Design review of the part shown in the three views and the two pictorial views. Dimensions are in mm from the part's minimum x, y and z. A direction names the side the tool comes from. Round coordinates to 2 decimals unless told otherwise and drop trailing zeros. Order: outer loops, then holes, each group sorted by start corner. A loop starts at its lowest first (then second) coordinate and runs counter-clockwise, first axis right, second up. Notation, with made-up numbers: M 84,87.5 L 101,87.5 A19 ccw 101,96.5 Z; hole C 15,-35.75 d9. An arc over 180 degrees is marked long. Write item = value, one per line. Start each with the question number.
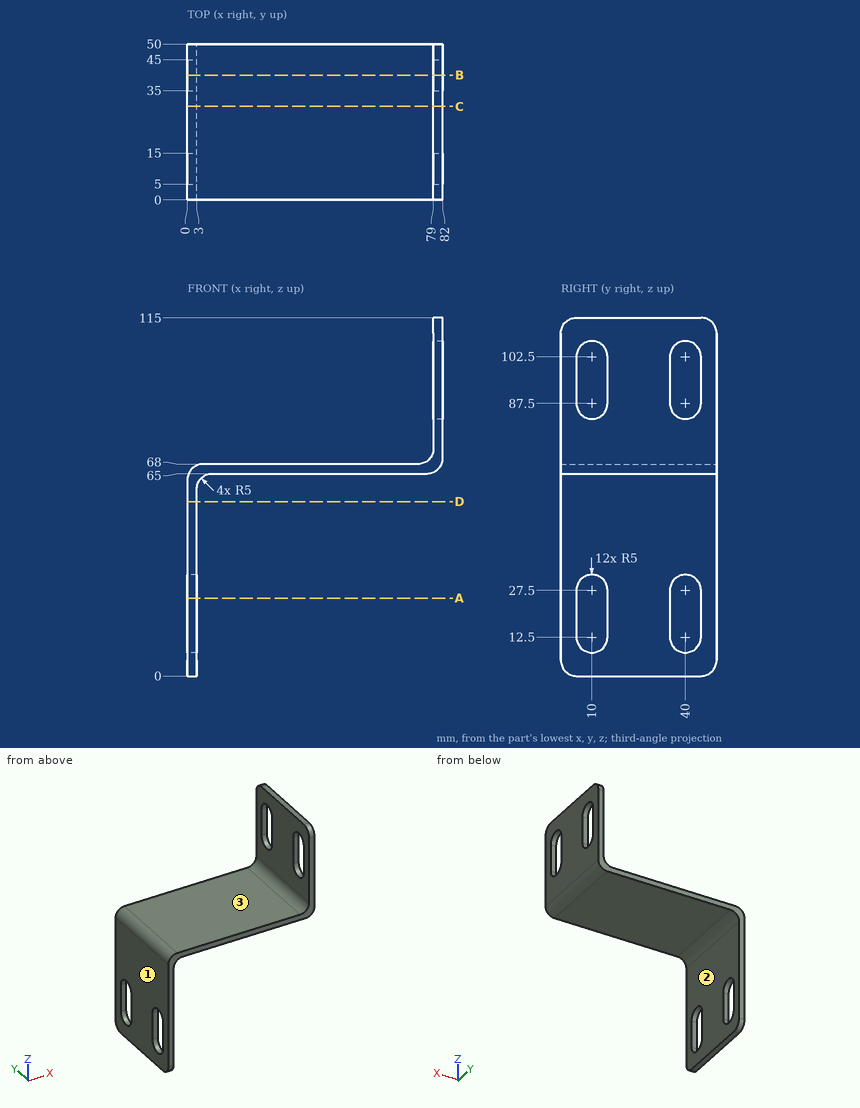
(1) For the marked faces 1, 2 and 3, list the 3-axis set-ups (+Z, -Z, +X, -X, +Y, -Y) from which the entire face can be reached by the end or side of a thin tool; tool diameter is ignored.
(2) For line 1 along X through (y, z) = (36, 41); line 2 along Z through (x, y) = (43.5, 47.5); line 3 along X through (y, z) = (31.5, 83), list the stretches that pass through material, from the lowest coordinate up.
(3) We need section B-B, the plane y = 40. Write out the cut boundary in (x, z).
(4) We need section A-A, the plane z = 25. Write out the cut boundary in (x, y), then the cut area to 3 significant figures.
(5) We need section D-D, the plane z = 56. Write out the cut boundary in (x, y).
(6) We need section C-C, the plane y = 30. Write out the cut boundary in (x, z), then the cut area to 3 significant figures.
(7) Insertion check: pin 1 (3 mm diameter, centred on x = 58, y = 6.5, fed in from +Z); pin 2 (15 mm diameter, centred on x = 48.5, y = 15, fed in from -Z); pin 3 (8 mm diameter, centred on y = 7, z = 99, fed in from -X). Each pin has a flat end and moves straight along its axis. Give the tip position at first contact, or say it passes through.
Values:
q1.face_1 = +Z, -Z, -X, +Y, -Y
q1.face_2 = -Z, +X, +Y, -Y
q1.face_3 = +Z, -X, +Y, -Y
q2.line_1 = 0 to 3
q2.line_2 = 65 to 68
q2.line_3 = 79 to 82
q3.outline = M 0,0 L 3,0 L 3,7.5 L 0,7.5 Z; M 0,32.5 L 3,32.5 L 3,60 A5 cw 8,65 L 77,65 A5 ccw 82,70 L 82,82.5 L 79,82.5 L 79,73 A5 cw 74,68 L 5,68 A5 ccw 0,63 Z; M 79,107.5 L 82,107.5 L 82,115 L 79,115 Z
q4.outline = M 0,0 L 3,0 L 3,5 L 0,5 Z; M 0,15 L 3,15 L 3,35 L 0,35 Z; M 0,45 L 3,45 L 3,50 L 0,50 Z
q4.area = 90.0 mm²
q5.outline = M 0,0 L 3,0 L 3,50 L 0,50 Z
q6.outline = M 0,0 L 3,0 L 3,60 A5 cw 8,65 L 77,65 A5 ccw 82,70 L 82,115 L 79,115 L 79,73 A5 cw 74,68 L 5,68 A5 ccw 0,63 Z
q6.area = 582 mm²
q7.pin_1 = 68
q7.pin_2 = 65
q7.pin_3 = 79
